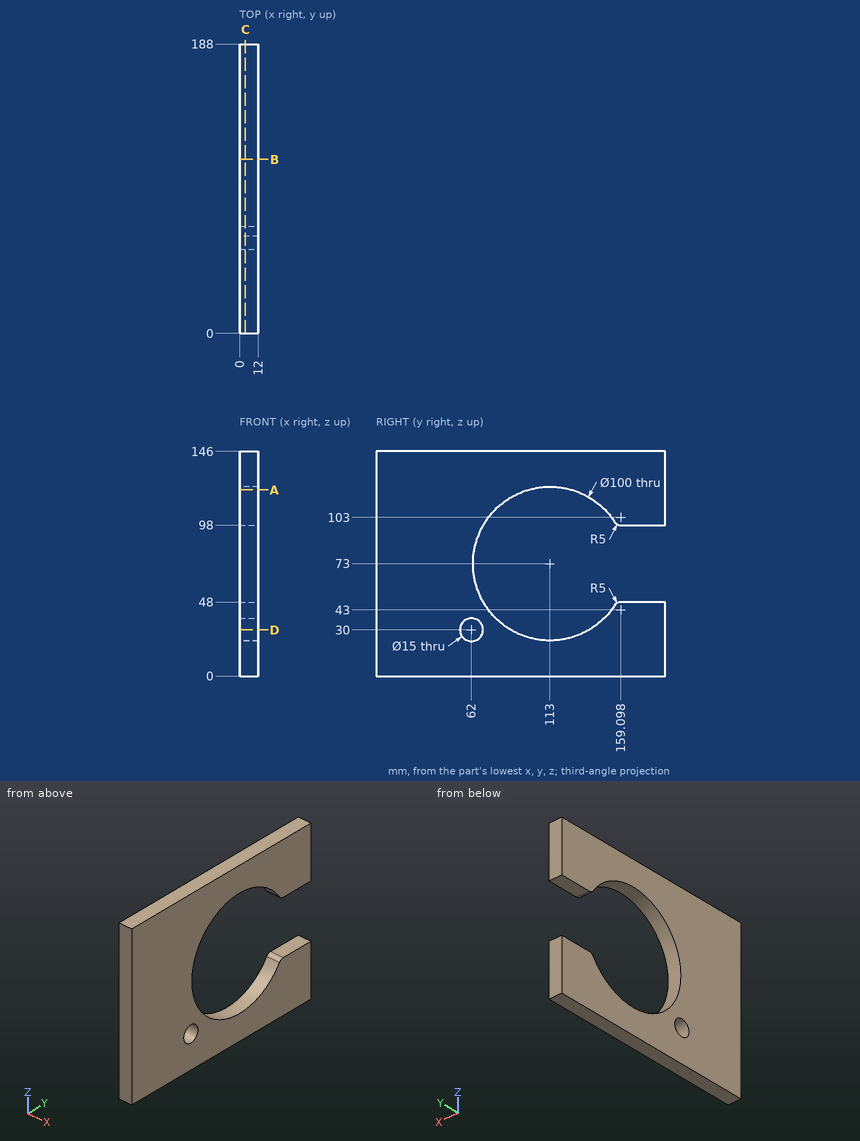
Verification items for this drawing (mm, ordinates from the low corner). Coordinates: 2 decimals unless noted, no trailing zeros. Write each loop counter-clockwise with the first axis right and the second up, starting at its lowest first coordinate (ties: lowest second). Pieces come first, ordered by that corner, then holes. Notation, with made-up numbers: M 71.5,4 L 105.5,4 A17 cw 105.5,34 Z; hole C 21.25,-15.75 d1. An arc over 180 degrees is marked long. One line per item, written item: value. Start each with the question number.
(1) Scan lines: line 1 along Z through (x, y) = (2.5, 113); line 2 along Z through (x, y) = (5, 179); line 3 along Y through (x, z) = (3, 30) (1 decimal). Record each from-to range of solid material in increasing order. Write a range as [from, to].
(2) Sectioned sample at C-C, the plane x = 3.75. Enter the section's corners in (y, z).
(3) Sectioned sample at A-A, the plane z = 121. Enter the section's corners in (x, y).
(4) Sectioned sample at B-B, the plane y = 113. Enter the section's corners in (x, z).
(5) Sectioned sample at D-D, the plane z = 30. Enter the section's corners in (x, y) (1 decimal), and give its area (3 significant figures).
(6) Depth check by flat-ended pin: pin 1 (4 mm diameter, centred on x = 1.5, z = 74.5, fed in from +Y). Enter the tip coordinate at first touch or a pass-through.
Filled sheet:
1. line 1: [0, 23], [123, 146]
1. line 2: [0, 48], [98, 146]
1. line 3: [0, 54.5], [69.5, 87.5], [138.5, 188]
2. outline: M 0,0 L 188,0 L 188,48 L 159.1,48 A5 ccw 154.91,45.73 A50 cw long 154.91,100.27 A5 ccw 159.1,98 L 188,98 L 188,146 L 0,146 Z; hole C 62,30 d15
3. outline: M 0,0 L 12,0 L 12,99 L 0,99 Z; M 0,127 L 12,127 L 12,188 L 0,188 Z
4. outline: M 0,0 L 12,0 L 12,23 L 0,23 Z; M 0,123 L 12,123 L 12,146 L 0,146 Z
5. outline: M 0,0 L 12,0 L 12,54.5 L 0,54.5 Z; M 0,69.5 L 12,69.5 L 12,87.5 L 0,87.5 Z; M 0,138.5 L 12,138.5 L 12,188 L 0,188 Z
5. area: 1,460 mm²
6. pin 1: y = 63.12
